Input: part model. Units: mm. Frame: model coordinates. A direction names the side the tool comes from. Coordinates: 2 decimals unless noted, no trailing zeros. Loops run counter-clockwise (first coordinate to the right, second up) from the corner with the lowest first, then second, coordinate; pieces in that order, holes last.
```python
from build123d import *

# Parameters (mm, degrees)
F1_DEPTH = 1.4
F2_SCALE = 1.25


# Not quite as in the source:
# - ends of sketch curves that miss each other by under 0.0002 mm in the source are joined


with BuildPart() as f1:
    # F0 (on Front) → F1 (new body)
    with BuildSketch(Plane.XZ):
        with BuildLine():
            Line((2.0343041438, 15.7069808039), (0.3523669438, 19.1131970039))
            Line((0.3523669438, 19.1131970039), (0.3523669438, -1.4730457961))
            Line((0.3523669438, -1.4730457961), (0.5645331438, -1.4730457961))
            Line((0.5645331438, -1.4730457961), (0.4553893438, 3.2909274039))
            ThreePointArc((0.4553893438, 3.2909274039), (0.5916556183, 3.5917542423), (0.9117258932, 3.6731219434))
            Line((0.9117258932, 3.6731219434), (5.3169493438, 2.7830798039))
            Line((5.3169493438, 2.7830798039), (4.8399119438, 3.7367228039))
            ThreePointArc((4.8399119438, 3.7367228039), (4.7582554065, 4.4182578922), (5.1286096155, 4.9961801528))
            Line((5.1286096155, 4.9961801528), (9.6409691438, 8.4717908039))
            Line((9.6409691438, 8.4717908039), (8.6805951438, 8.9006952039))
            ThreePointArc((8.6805951438, 8.9006952039), (8.4915257857, 9.0857200238), (8.4685111742, 9.3492575516))
            Line((8.4685111742, 9.3492575516), (9.2975103438, 12.3747294039))
            Line((9.2975103438, 12.3747294039), (6.6119175438, 11.9498382039))
            ThreePointArc((6.6119175438, 11.9498382039), (6.3606002996, 11.996951044), (6.1956594084, 12.1923309026))
            Line((6.1956594084, 12.1923309026), (5.8086171438, 13.2239784039))
            Line((5.8086171438, 13.2239784039), (3.7461117438, 10.8478846039))
            ThreePointArc((3.7461117438, 10.8478846039), (3.1301426273, 10.7291430881), (2.8684469448, 11.2992470593))
            Line((2.8684469448, 11.2992470593), (4.0912977438, 16.4041346039))
            Line((4.0912977438, 16.4041346039), (2.5628527438, 15.5436588039))
            ThreePointArc((2.5628527438, 15.5436588039), (2.2634525656, 15.511644492), (2.0343041438, 15.7069808039))
        make_face()
        with BuildLine():
            Line((0.3523669438, -1.4730457961), (0.3523669438, 19.1131970039))
            Line((0.3523669438, 19.1131970039), (-1.3295956562, 15.7069808039))
            ThreePointArc((-1.3295956562, 15.7069808039), (-1.5587335044, 15.5116477594), (-1.858122509, 15.5436523149))
            Line((-1.858122509, 15.5436523149), (-3.3865892562, 16.4041346039))
            Line((-3.3865892562, 16.4041346039), (-2.1637316562, 11.2992426039))
            ThreePointArc((-2.1637316562, 11.2992426039), (-2.4254367706, 10.7291417351), (-3.0413892842, 10.8478967322))
            Line((-3.0413892842, 10.8478967322), (-5.1039086562, 13.2239784039))
            Line((-5.1039086562, 13.2239784039), (-5.4909284562, 12.1923320039))
            ThreePointArc((-5.4909284562, 12.1923320039), (-5.6558664119, 11.996951044), (-5.9071825723, 11.9498450545))
            Line((-5.9071825723, 11.9498450545), (-8.5927764562, 12.3747294039))
            Line((-8.5927764562, 12.3747294039), (-7.7637966562, 9.3492592039))
            ThreePointArc((-7.7637966562, 9.3492592039), (-7.786817298, 9.0857200238), (-7.9758860019, 8.9006937389))
            Line((-7.9758860019, 8.9006937389), (-8.9362606562, 8.4717908039))
            Line((-8.9362606562, 8.4717908039), (-4.4238744562, 4.9961818039))
            ThreePointArc((-4.4238744562, 4.9961818039), (-4.0535446709, 4.4182480852), (-4.1352063244, 3.7367242387))
            Line((-4.1352063244, 3.7367242387), (-4.6122408562, 2.7830798039))
            Line((-4.6122408562, 2.7830798039), (-0.2070172562, 3.6731212039))
            ThreePointArc((-0.2070172562, 3.6731212039), (0.1130528694, 3.5917542423), (0.2493205388, 3.2909273719))
            Line((0.2493205388, 3.2909273719), (0.1401753438, -1.4730457961))
            Line((0.1401753438, -1.4730457961), (0.3523669438, -1.4730457961))
        make_face()
    extrude(amount=F1_DEPTH)


with BuildPart() as f1_1:
    # F2: moved
    add(f1.part.scale(F2_SCALE).moved(Location((-0.088091736, 0.35, -4.778299251))))


solid = f1_1.part
```
Item 1: Section query D-D (z = 8.25). Output: boundary loops of the cut face in (x, y).
Result:
outline: (-10.16, -1.4) - (10.87, -1.4) - (10.87, 0.35) - (-10.16, 0.35) - close
Item 2: Reachability of faces 1 (the face through (-5.551, -0.513, -0.695)), 2 (the face through (-3.568, -0.513, 12.581)), 3 (the face through (11.008, -0.513, 8.773)), 4 (the face through (-0.684, -0.513, 17.014)), 5 (the face through (0, 0.35, 6)) from +Z, -Z, +X, -X, +Y, -Y: full face, straight path, thin tool, end or side. Return the list, or none.
Result:
face 1: -X, +Y, -Y
face 2: +Y, -Y
face 3: +X, +Y, -Y
face 4: +Z, +Y, -Y
face 5: +Z, -Z, +X, -X, +Y
Item 3: Section query C-C (z = 15.25). Output: boundary loops of the cut face in (x, y).
Result:
outline: (-4.21, -1.4) - (-3.47, -1.4) - (-3.47, 0.35) - (-4.21, 0.35) - close; (-1.56, -1.4) - (2.26, -1.4) - (2.26, 0.35) - (-1.56, 0.35) - close; (4.18, -1.4) - (4.91, -1.4) - (4.91, 0.35) - (4.18, 0.35) - close
Item 4: Section query A-A (z = 11.25). Output: boundary loops of the cut face in (x, y), then the cut area to 3 significant figures.
Result:
outline: (-6.66, -1.4) - (-6.03, -1.4) - (-6.03, 0.35) - (-6.66, 0.35) - close; (-3.25, -1.4) - (3.95, -1.4) - (3.95, 0.35) - (-3.25, 0.35) - close; (6.74, -1.4) - (7.36, -1.4) - (7.36, 0.35) - (6.74, 0.35) - close
area: 14.8 mm2
Item 5: Mould query, pull axis Z, two halves, no side actions, for faces 6 (the face through (3.766, -0.513, -0.735)), 7 (the face through (4.084, -0.513, 15.197)), 8 (the face through (11.371, -0.513, 6.076)). Classes: +Z half, -Z half, draft (parallel to the pull), parting line (faces both ways), or undercut.
Result:
face 6: -Z half
face 7: +Z half
face 8: undercut
Item 6: Section query B-B (x = 8.5). Output: boundary loops of the cut face in (y, z).
Result:
outline: (-1.4, 3.14) - (0.35, 3.14) - (0.35, 10.21) - (-1.4, 10.21) - close
Item 7: Contact query for flat-ended pins moving along their axis: P1, Ø1, axis at x = -0.5, y = -0.5, coming from the -Z side; P2, Ø1, axis at y = -0.5, z = 9, coming from the -X side; P3, Ø1, axis at x = 2.5, y = -1, coming from the -Z side. Output: stop coordinate, or through.
Result:
P1: stops at z = -0.32
P2: stops at x = -10.5
P3: stops at z = -0.58
Item 8: Line query: L1, parallel to Z at x = -5.75, y = -1.2; L2, parallel to X at y = 0, z = 14; L3, parallel to X at y = -0.6, z = 0. Output: solid intervals per line, ascending.
Result:
L1: z = -1.28 to -1.09, 1.57 to 10.92
L2: x = -3.91 to 4.61
L3: x = -5.21 to 5.91
